```python
from build123d import *

# Parameters (mm, degrees)
SKETCH1_W               = 75
SKETCH1_H               = 75
BOSS_EXTRUDE1_DEPTH     = 24
SKETCH2_W               = 20
SKETCH2_H               = 19
CUT_EXTRUDE1_DEPTH      = 45
SKETCH3_W               = 19
SKETCH3_H               = 20
CUT_EXTRUDE2_DEPTH      = 45
CUT_EXTRUDE3_DEPTH      = 109.747413762
CUT_EXTRUDE3_DEPTH_BACK = 109.747413762
SKETCH4_W               = 45
SKETCH4_H               = 45
FILLET1_R               = 5
CHAMFER1_SIZE           = 10
SKETCH5_W               = 29
SKETCH5_H               = 8
BOSS_EXTRUDE2_DEPTH     = 37.5
SKETCH6_R               = 11.5
CUT_EXTRUDE4_DEPTH      = 7
FILLET2_R               = 5
CHAMFER3_SIZE           = 5
CUT_EXTRUDE5_DEPTH      = 93.146622293
CUT_EXTRUDE5_DEPTH_BACK = 93.146622293
SKETCH7_R               = 2.65
CUT_EXTRUDE6_DEPTH      = 105.986903945
CUT_EXTRUDE6_DEPTH_BACK = 105.986903945
SKETCH8_R               = 2.65
SKETCH9_R               = 2.65
CUT_EXTRUDE7_DEPTH      = 10
SKETCH10_R              = 2.65
CUT_EXTRUDE8_DEPTH      = 10
CUT_EXTRUDE12_DEPTH     = 19
CUT_EXTRUDE13_REACH     = 111.959
CUT_EXTRUDE14_REACH     = 140.283
SKETCH14_R              = 10
CUT_EXTRUDE15_DEPTH     = 10
CHAMFER5_SIZE           = 4
CHAMFER6_SIZE           = 1
CHAMFER8_SIZE2          = 0.550911948
CHAMFER8_SIZE           = 7


with BuildPart() as part:
    # Sketch1 → Boss-Extrude1 (new body)
    with BuildSketch(Plane.XY):
        with Locations((37.5, 37.5)):
            Rectangle(SKETCH1_W, SKETCH1_H)
    extrude(amount=BOSS_EXTRUDE1_DEPTH)

    # Sketch2 → Cut-Extrude1 (cut)
    with BuildSketch(Plane.XZ):
        with Locations((15, 14.5)):
            Rectangle(SKETCH2_W, SKETCH2_H)
    extrude(amount=-CUT_EXTRUDE1_DEPTH, mode=Mode.SUBTRACT)

    # Sketch3 → Cut-Extrude2 (cut)
    with BuildSketch(Plane(origin=(75, 0, 0), x_dir=(0, 0, -1), z_dir=(1, 0, 0))):
        with Locations((-14.5, 60)):
            Rectangle(SKETCH3_W, SKETCH3_H)
    extrude(amount=-CUT_EXTRUDE2_DEPTH, mode=Mode.SUBTRACT)

    # Sketch4 → Cut-Extrude3 (cut, two sides: drawn at the far end of the back side and taken through both)
    with BuildSketch(Plane.XY.offset(24).offset(-CUT_EXTRUDE3_DEPTH_BACK)):
        with Locations((52.5, 22.5)):
            Rectangle(SKETCH4_W, SKETCH4_H)
    extrude(amount=CUT_EXTRUDE3_DEPTH + CUT_EXTRUDE3_DEPTH_BACK, mode=Mode.SUBTRACT)

    # Fillet1
    fillet1_edges = [part.edges().sort_by_distance(p)[0] for p in [
        (0, 75, 12),
    ]]
    fillet(fillet1_edges, radius=FILLET1_R)

    # Chamfer1
    chamfer1_edges = [part.edges().sort_by_distance(p)[0] for p in [
        (30, 45, 12),
    ]]
    chamfer(chamfer1_edges, length=CHAMFER1_SIZE)

    # Sketch5 → Boss-Extrude2 (add)
    with BuildSketch(Plane.ZY):
        with Locations((14.5, 41)):
            Rectangle(SKETCH5_W, SKETCH5_H)
    extrude(amount=BOSS_EXTRUDE2_DEPTH)

    # Sketch6 → Cut-Extrude4 (cut)
    with BuildSketch(Plane(origin=(0, 45, 0), x_dir=(1, 0, 0), z_dir=(0, 1, 0))):
        with Locations(Location((-21, -15.000000001, 0), (0, 0, 180))):
            Circle(SKETCH6_R)
    extrude(amount=-CUT_EXTRUDE4_DEPTH, mode=Mode.SUBTRACT)

    # Fillet2
    fillet2_edges = [part.edges().sort_by_distance(p)[0] for p in [
        (-37.5, 41, 29),
        (-37.5, 41, 0),
    ]]
    fillet(fillet2_edges, radius=FILLET2_R)

    # Chamfer3
    chamfer3_edges = [part.edges().sort_by_distance(p)[0] for p in [
        (0, 45, 12),
        (0, 37, 12),
    ]]
    chamfer(chamfer3_edges, length=CHAMFER3_SIZE)

    # Sketch7 → Cut-Extrude5 (cut, two sides: drawn at the far end of the back side and taken through both)
    with BuildSketch(Plane.XZ.offset(-45).offset(-CUT_EXTRUDE5_DEPTH_BACK)):
        with Locations((59, 15)):
            Circle(SKETCH7_R)
    extrude(amount=CUT_EXTRUDE5_DEPTH + CUT_EXTRUDE5_DEPTH_BACK, mode=Mode.SUBTRACT)

    # Sketch8 → Cut-Extrude6 (cut, two sides: drawn at the far end of the back side and taken through both)
    with BuildSketch(Plane(origin=(30, 0, 0), x_dir=(0, 0, -1), z_dir=(1, 0, 0)).offset(-CUT_EXTRUDE6_DEPTH_BACK)):
        with Locations((-15, 16)):
            Circle(SKETCH8_R)
    extrude(amount=CUT_EXTRUDE6_DEPTH + CUT_EXTRUDE6_DEPTH_BACK, mode=Mode.SUBTRACT)

    # Sketch9 → Cut-Extrude7 (cut)
    with BuildSketch(Plane.XY.offset(5)):
        with Locations((15, 22.5)):
            Circle(SKETCH9_R)
    extrude(amount=-CUT_EXTRUDE7_DEPTH, mode=Mode.SUBTRACT)

    # Sketch10 → Cut-Extrude8 (cut)
    with BuildSketch(Plane.XY.offset(5)):
        with Locations((52.5, 60)):
            Circle(SKETCH10_R)
    extrude(amount=-CUT_EXTRUDE8_DEPTH, mode=Mode.SUBTRACT)

    # Sketch11 → Cut-Extrude12 (cut)
    with BuildSketch(Plane.XY.offset(24)):
        Polygon((34, 70), (30, 71), (30, 70), align=None)
        Polygon((30, 50), (34, 50), (30, 49), align=None)
        Polygon((26, 45), (25, 41), (25, 45), align=None)
        Polygon((5, 45), (4, 45), (5, 41), align=None)
    extrude(amount=-CUT_EXTRUDE12_DEPTH, mode=Mode.SUBTRACT)

    # Cut-Extrude13: up to this face of the body (flat: up to its plane)
    cut_extrude13_end = Plane(part.part.faces().sort_by_distance((15, 45, 14.5))[0])
    # Sketch12 → Cut-Extrude13 (cut, up to the picked face)
    with BuildSketch(Plane.XZ, mode=Mode.PRIVATE) as cut_extrude13_sk1:
        Polygon((5, 5), (4, 5), (5, 9), align=None)
    cut_extrude13_tool1 = split(extrude(cut_extrude13_sk1.sketch, amount=-CUT_EXTRUDE13_REACH, mode=Mode.PRIVATE), bisect_by=cut_extrude13_end, keep=Keep.BOTH, mode=Mode.PRIVATE)
    # Sketch12 → Cut-Extrude13 (cut, up to the picked face)
    with BuildSketch(Plane.XZ, mode=Mode.PRIVATE) as cut_extrude13_sk2:
        Polygon((25, 5), (26, 5), (25, 9), align=None)
    cut_extrude13_tool2 = split(extrude(cut_extrude13_sk2.sketch, amount=-CUT_EXTRUDE13_REACH, mode=Mode.PRIVATE), bisect_by=cut_extrude13_end, keep=Keep.BOTH, mode=Mode.PRIVATE)
    add(cut_extrude13_tool1.solids().sort_by(Axis((4.666667, 0, 6.333333), (0, 1, 0)))[0], mode=Mode.SUBTRACT)
    add(cut_extrude13_tool2.solids().sort_by(Axis((25.333333, 0, 6.333333), (0, 1, 0)))[0], mode=Mode.SUBTRACT)

    # Cut-Extrude14: up to this face of the body (flat: up to its plane)
    cut_extrude14_end = Plane(part.part.faces().sort_by_distance((30, 60, 14.5))[0])
    # Sketch13 → Cut-Extrude14 (cut, up to the picked face)
    with BuildSketch(Plane(origin=(75, 0, 0), x_dir=(0, 0, -1), z_dir=(1, 0, 0)), mode=Mode.PRIVATE) as cut_extrude14_sk1:
        Polygon((-5, 50), (-5, 49), (-9, 50), align=None)
    cut_extrude14_tool1 = split(extrude(cut_extrude14_sk1.sketch, amount=-CUT_EXTRUDE14_REACH, mode=Mode.PRIVATE), bisect_by=cut_extrude14_end, keep=Keep.BOTH, mode=Mode.PRIVATE)
    # Sketch13 → Cut-Extrude14 (cut, up to the picked face)
    with BuildSketch(Plane(origin=(75, 0, 0), x_dir=(0, 0, -1), z_dir=(1, 0, 0)), mode=Mode.PRIVATE) as cut_extrude14_sk2:
        Polygon((-5, 70), (-5, 71), (-9, 70), align=None)
    cut_extrude14_tool2 = split(extrude(cut_extrude14_sk2.sketch, amount=-CUT_EXTRUDE14_REACH, mode=Mode.PRIVATE), bisect_by=cut_extrude14_end, keep=Keep.BOTH, mode=Mode.PRIVATE)
    add(cut_extrude14_tool1.solids().sort_by(Axis((75, 49.666667, 6.333333), (-1, 0, 0)))[0], mode=Mode.SUBTRACT)
    add(cut_extrude14_tool2.solids().sort_by(Axis((75, 70.333333, 6.333333), (-1, 0, 0)))[0], mode=Mode.SUBTRACT)

    # Sketch14 → Cut-Extrude15 (cut)
    with BuildSketch(Plane(origin=(0, 38, 0), x_dir=(1, 0, 0), z_dir=(0, 1, 0))):
        with Locations(Location((-21, -15.000000001, 0), (0, 0, 180))):
            Circle(SKETCH14_R)
    extrude(amount=-CUT_EXTRUDE15_DEPTH, mode=Mode.SUBTRACT)

    # Chamfer5
    chamfer5_edges = [part.edges().sort_by_distance(p)[0] for p in [
        (0, 41, 24),
    ]]
    chamfer(chamfer5_edges, length=CHAMFER5_SIZE)

    # Chamfer6
    chamfer6_edges = [part.edges().sort_by_distance(p)[0] for p in [
        (0, 41, 29),
    ]]
    chamfer(chamfer6_edges, length=CHAMFER6_SIZE - 0.0001)  # a hair under: the kernel refuses the full size

    # Chamfer8
    chamfer8_edges = [part.edges().sort_by_distance(p)[0] for p in [
        (-9.5, 38, 15.000000001),
    ]]
    chamfer8_side = [part.faces().sort_by_distance(p)[0] for p in [
        (-9.5, 38.011018239, 15.000000001),
    ]]
    chamfer(chamfer8_edges, length=CHAMFER8_SIZE - 0.0001, length2=CHAMFER8_SIZE2 - 0.0001, reference=chamfer8_side[0])  # a hair under: the kernel refuses the full size


with BuildPart() as body_2:
    # Mirror1: mirrored copy
    add(part.part.mirror(Plane(origin=(75, 0, 24), x_dir=(0, 0, 1), z_dir=(-1, 0, 0))))


solid = body_2.part
```
Could you check a few things on this model? Use its own coordinates, in mm. A direction names the side the tool comes from. Round coordinates to 2 decimals unless told otherwise and drop trailing zeros. Order: outer loops, then holes, each group sorted by start corner. A loop starts at its lowest first (then second) coordinate and runs counter-clockwise, first axis right, second up. Notation, with made-up numbers: (-24, -17) -> (-17, -17) arc R21 ccw to (-17, 3) -> close; hole circle Ø9 at (79.25, 78.25). An arc over 180 degrees is marked (long way). One line per question, with ' | ' between items.
Q1. If we section it at C-C on y = 47: Write out the boundary of the cut face in (x, z).
Computed values:
outline: (75, 0) -> (153, 0) -> (153, 24) -> (75, 24) -> close; hole circle Ø5.3 at (91, 15)
Q2. If I drill on line 1 (Z direction, x = 171, y = 37.85); line 2 (Y direction, x = 135, z = 3.65); line 3 (X direction, y = 29, z = 23.75), over which ranges is the centre line in solid material (lowest first)? Write a range as from..to.
Computed values:
line 1: 0..5, 25..29 | line 2: 0..19.85, 25.15..75 | line 3: 120..125, 145..150
Q3. I'm going to push flat-ended pins straight in: pin 1 (12 mm diameter, centred on x = 87, z = 12, fed in from -Y); pin 2 (2 mm diameter, centred on y = 20, z = 12, fed in from +X); pin 3 (17.5 mm diameter, centred on x = 91.5, y = 58.5, fed in from +Z). Where does each tip first touch, or does it pass through?
Computed values:
pin 1: y = 45 | pin 2: x = 150 | pin 3: z = 24
Q4. Which directions (+Z, -Z, +X, -X, +Y, -Y) give clear straight access to the entire face, cutting with the end or side of a thin tool? Please do faces 1 (the face through (145.5, 22.2, 7)), 2 (the face through (145.5, 43, 14.6)), 3 (the face through (116, 45, 0)), 4 (the face through (176, 38, 6)).
Computed values:
face 1: -Y | face 2: +Z | face 3: -Z, +X, -X, +Y, -Y | face 4: +Y
Q5. If we section it at B-B on x = 97.5: Write out the boundary of the cut face in (y, z), plus the area to 4 significant figures.
Computed values:
outline: (45, 0) -> (57.35, 0) -> (57.35, 5) -> (49, 5) -> (50, 9) -> (50, 24) -> (45, 24) -> close; (62.65, 0) -> (75, 0) -> (75, 24) -> (70, 24) -> (70, 9) -> (71, 5) -> (62.65, 5) -> close | area: 309.5 mm²
Q6. We'd pull the mould along Z, two halves only. Please class faces 5 (the face through (95, 70, 17)), 6 (the face through (122.54, 14.99, 12.55)), 7 (the face through (148, 41, 26)): released by +Z, released by -Z, zero draft, split by the parting line, or undercut.
Computed values:
face 5: zero draft | face 6: undercut | face 7: released by +Z
Q7. If we section it at A-A on y = 16: Write out the boundary of the cut face in (x, z).
Computed values:
outline: (120, 0) -> (150, 0) -> (150, 12.35) -> (145, 12.35) -> (145, 9) -> (146, 5) -> (124, 5) -> (125, 9) -> (125, 12.35) -> (120, 12.35) -> close; (120, 17.65) -> (125, 17.65) -> (125, 24) -> (120, 24) -> close; (145, 17.65) -> (150, 17.65) -> (150, 24) -> (145, 24) -> close
Q8. If we section it at D-D on x = 86: Write out the boundary of the cut face in (y, z).
Computed values:
outline: (45, 0) -> (75, 0) -> (75, 24) -> (70, 24) -> (70, 9) -> (71, 5) -> (49, 5) -> (50, 9) -> (50, 24) -> (45, 24) -> close
